For this review, use the dimensioned drawing (mm, ordinates from the lowest corner) and the shaded views. Give positions to 0.01 mm unless a question says otherwise; leave off trailing zeros. Order: outer loops, then holes, each group sorted by start corner. A loop starts at its lowest first (then second) coordinate and runs counter-clockwise, first axis right, second up. Notation, with made-up numbers: (-7.5, -29) - (35.5, -29) arc R8 cw to (35.5, -20) - close; hole circle Ø8 at (24.5, 30.5). An arc over 180 degrees is marked (long way). Use a Markdown table: item, result. Add a question column.
1) Clearance check with flat-ended pins moving along their axes: P1, Ø1.9, axis at y = 2.5, z = 38, coming from the -X side; P2, Ø3, axis at x = 10.5, y = 5, coming from the +Z side; P3, Ø1.7, axis at x = 12.5, y = 2, coming from the -Z side. State where each tip first meets the part, or that it passes through.
2) We need section C-C on z = 38.1. Write out the cut boundary in (x, y), then the cut area to 3 significant figures.
3) Wall thickness on L1, parallel to X at y = 1.5, z = 38.1; L2, parallel to X at y = 4.75, z = 6.5; L3, parallel to X at y = 1.5, z = 44 (1 decimal): over which ranges is each line inside the solid? List them lowest first.
4) We need section A-A on z = 60.5. Write out the cut boundary in (x, y), then the cut area to 3 significant figures.
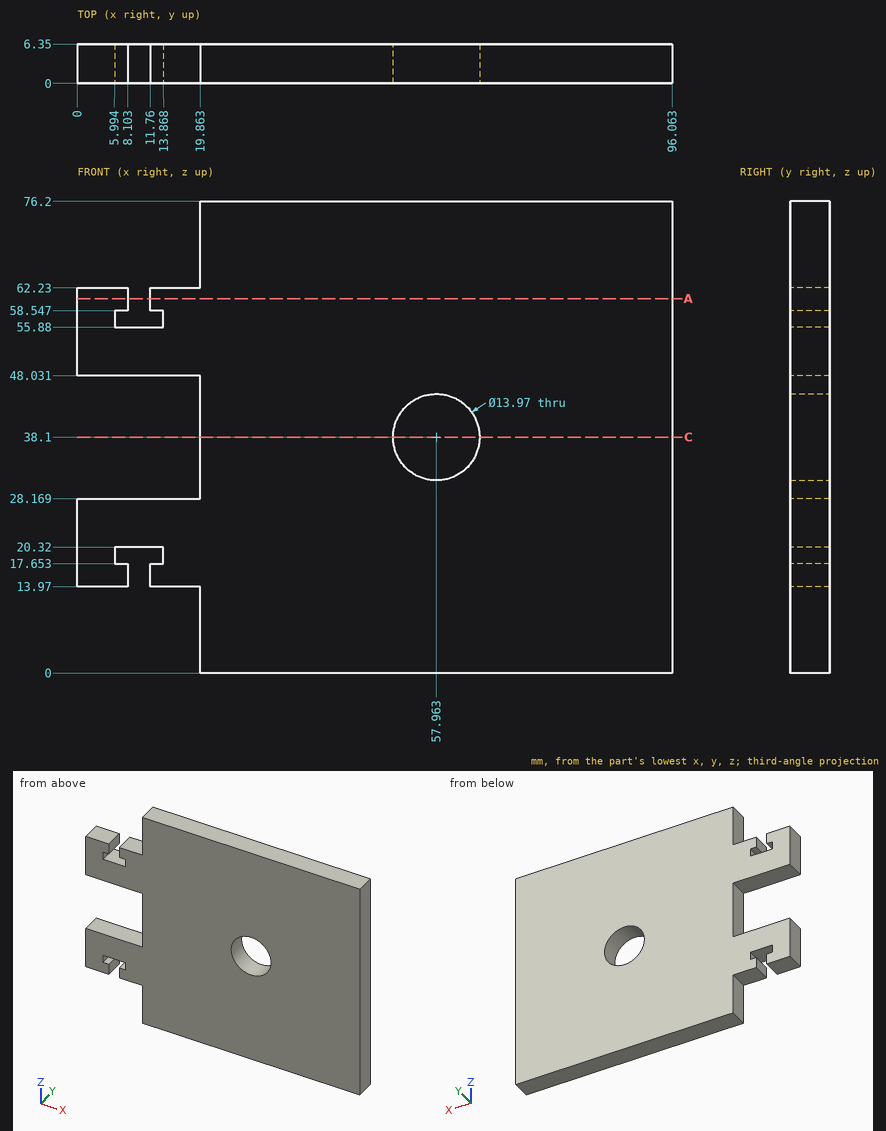
Checked values:
| question | item | result |
|---|---|---|
| 1 | P1 | x = 19.86 |
| 1 | P2 | z = 62.23 |
| 1 | P3 | z = 13.97 |
| 2 | outline | (19.86, 0) - (50.98, 0) - (50.98, 6.35) - (19.86, 6.35) - close; (64.95, 0) - (96.06, 0) - (96.06, 6.35) - (64.95, 6.35) - close |
| 2 | area | 395 mm² |
| 3 | L1 | 19.86 to 50.98, 64.95 to 96.06 |
| 3 | L2 | 19.86 to 96.06 |
| 3 | L3 | 19.9 to 54.2, 61.7 to 96.1 |
| 4 | outline | (0, 0) - (8.1, 0) - (8.1, 6.35) - (0, 6.35) - close; (11.76, 0) - (96.06, 0) - (96.06, 6.35) - (11.76, 6.35) - close |
| 4 | area | 587 mm² |
